Can you work these out from the model? Positions are in its coordinate system, mm. A direction names the side the tool comes from. Give positions to 0.01 mm unless a question says otherwise; leave off trailing zeros. Write each loop counter-clockwise with the first axis right and the second up, starting at its lowest first coordinate (ties: lowest second). Pieces come first, ordered by that corner, then holes.
1. Suppose I cut it at C-C (z = 41.5). Please give me the cut outline in (x, y), and give its area (3 significant figures).
2. Suppose I cut it at D-D (z = 60.5). Please give me the cut outline in (x, y).
3. If I drill on probe 1 along Z at (x, y) = (0, 6); probe 2 along Y at (x, z) = (0, 47); probe 3 along Z at (x, y) = (-21.5, 4), over which ranges is the centre line in solid material (lowest first)?
4. Thinking about a two-plate mould opening in X: for faces 1 (the flat face through (-1.5, -11, 26)), 2 (the cylindrical face through (-3.34, -25.43, 7.18)), 3 (the cylindrical face through (0.3, 7.57, 11.496)), 4 (the cylindrical face through (0, 7.6, 61.5)), which applies, pulls with the +X half, pulls with the -X half, needs draft (parallel to the pull), parting line crosses it, or undercut?
5. On a 3-axis mill with a long thin cutter (end or side, diameter ignored), from which of +Z, -Z, +X, -X, +Y, -Y can I reach the whole of each face in a straight line? I mean faces 5 (the cylindrical face through (4.5, 8.65, 43.07)), 6 (the cylindrical face through (5.66, 7.94, 12.39)), 7 (the flat face through (1.5, 11, 26)), 8 (the flat face through (0, -9, 25.901)), 9 (the flat face through (-11.95, 0, 27)). Say none if no direction works.
6. Suppose I cut it at B-B (y = 17). Please give me the cut outline in (x, z), and give its area (3 significant figures).
7. I'm going to push flat-ended pins straight in: pin 1 (0.9 mm diameter, centred on x = -0.5, z = 17.5, fed in from -Y); pin 2 (1.5 mm diameter, centred on x = 0.5, z = 26.5, fed in from +Y); pin 3 (10 mm diameter, centred on y = 13.5, z = 20.5, fed in from -X). Where does each tip first touch, or does it pass through?
8. Suppose I cut it at A-A (x = 22.5). Please give me the cut outline in (y, z).
Solid Edge part; units mm, degrees
sketch "Sketch1" plane through (0, 0, 0) normal (0, 0, 1) x (1, 0, 0)
  circle A0 centre (0, 0) radius 9.75
extrude "ProtrusioneEstrusa_1" add sketch "Sketch1" along normal blind 67
sketch "Sketch2" plane through (0, 0, 6.1) normal (0, 0, -1) x (1, 0, 0)
  circle A0 centre (0, 0) radius 25.65
extrude "ProtrusioneEstrusa_2" add sketch "Sketch2" against normal blind 2.2
sketch "Sketch3" plane through (0, 0, 16.6) normal (0, 0, 1) x (1, 0, 0)
  circle A0 centre (0, 0) radius 25.65
extrude "ProtrusioneEstrusa_3" add sketch "Sketch3" along normal blind 3.2
sketch "Sketch4" plane through (0, 0, 19.8) normal (0, 0, 1) x (1, 0, 0)
  line L0 (-11.95, -1.5) -> (-9.6339, -1.5)
  line L1 (-9.6339, -1.5) -> (-9.6339, 1.5)
  line L2 (-11.95, 1.5) -> (-9.6339, 1.5)
  line L3 (-11.95, 0) -> (-11.95, 1.5)
  line L4 (-11.95, 0) -> (-11.95, -1.5)
  line L5 (0, -11.95) -> (1.5, -11.95)
  line L6 (1.5, -11.95) -> (1.5, -9.6339)
  line L7 (1.5, -9.6339) -> (-1.5, -9.6339)
  line L8 (-1.5, -11.95) -> (-1.5, -9.6339)
  line L9 (0, -11.95) -> (-1.5, -11.95)
  line L10 (1.5, 11.95) -> (1.5, 9.6339)
  line L11 (-1.5, 9.6339) -> (1.5, 9.6339)
  line L12 (-1.5, 11.95) -> (-1.5, 9.6339)
  line L13 (0, 11.95) -> (-1.5, 11.95)
  line L14 (0, 11.95) -> (1.5, 11.95)
  line L15 (11.95, 0) -> (11.95, -1.5)
  line L16 (11.95, -1.5) -> (9.6339, -1.5)
  line L17 (9.6339, 1.5) -> (9.6339, -1.5)
  line L18 (11.95, 1.5) -> (9.6339, 1.5)
  line L19 (11.95, 0) -> (11.95, 1.5)
extrude "ProtrusioneEstrusa_4" add sketch "Sketch4" along normal blind 15
sketch "Sketch5" plane through (0, 5.45, 33.5) normal (0, -1, 0) x (0, 0, -1)
  circle A0 centre (21.05, 0) radius 1
  circle A1 centre (-27, 0) radius 1
extrude "ScavoEstrusione_3" cut sketch "Sketch5" against normal blind 12.2631 and the other way blind 0.5254
sketch "Sketch6" plane through (0, 0, 0) normal (0, 0, -1) x (1, 0, 0)
  line L0 (3.6239, 9.0515) -> (3.6239, 6.1055)
  arc A0 (-3.6239, 6.1055) -> (3.6239, 6.1055) centre (0, 0) cw
  line L1 (-3.6239, 9.0515) -> (-3.6239, 6.1055)
  line L2 (-3.6239, 9.0515) -> (3.6239, 9.0515)
extrude "ProtrusioneEstrusa_5" add sketch "Sketch6" along normal blind 6
sketch "Sketch7" plane through (0, 0.3492, 0) normal (0, 0, -1) x (0, -1, 0)
  circle A0 centre (0.3492, 0) radius 10.346
extrude "ProtrusioneEstrusa_6" add sketch "Sketch7" against normal blind 6.5682
sketch "Sketch8" plane through (0, 0, 0) normal (0, 0, 1) x (1, 0, 0)
  line L0 (-1.5, 6.9397) -> (-1.5, 5.45)
  line L1 (-1.5, 5.45) -> (1.5, 5.45)
  line L2 (1.5, 5.45) -> (1.5, 6.9397)
  arc A0 (1.5, 6.9397) -> (-1.5, 6.9397) centre (0, 0) cw
extrude "ScavoEstrusione_1" cut sketch "Sketch8" along normal mid plane 447.4642
fillet "Rotondo_1" radius 1.5 1 edges at (-1.5, -10.792, 34.8)
fillet "Rotondo_2" radius 1.5 1 edges at (1.5, -10.792, 34.8)
fillet "Rotondo_3" radius 1.5 3 edges at (-10.792, -1.5, 34.8) (-1.5, 10.792, 34.8) (10.792, 1.5, 34.8)
fillet "Rotondo_4" radius 1.5 3 edges at (-10.792, 1.5, 34.8) (1.5, 10.792, 34.8) (10.792, -1.5, 34.8)
sketch "Sketch9" plane through (0, 0, 0) normal (0, 0, -1) x (1, 0, 0)
  circle A0 centre (0, 8.7109) radius 1.2
extrude "ScavoEstrusione_5" cut sketch "Sketch9" along normal up to vertex (6 mm away) and the other way blind 25.9007
sketch "Sketch10" plane through (0, 0, 8.3) normal (0, 0, 1) x (-1, 0, 0)
  arc A0 (-1.6217, 9.6142) -> (1.6217, 9.6142) centre (0, 0) cw
  line L0 (1.1232, 8.2885) -> (1.6217, 9.6142)
  line L1 (-1.1232, 8.2885) -> (-1.6217, 9.6142)
  arc A1 (1.1232, 8.2885) -> (-1.1232, 8.2885) centre (0, 8.7109) cw
extrude "Cutout1" cut sketch "Sketch10" along normal up to vertex (8.3 mm away)
sketch "Sketch11" plane through (-2.3873, -9.0515, -3) normal (0, -1, 0) x (0, 0, 1)
  line L0 (-3, -3.3873) -> (-3, -1.3873)
  line L1 (-0.9394, -1.7204) -> (-3, -1.3873)
  arc A0 (-0.9394, -1.7204) -> (-0.7687, -1.667) centre (-0.9074, -1.523) ccw
  arc A1 (-0.94, -3.0543) -> (-0.7683, -3.1079) centre (-0.9078, -3.2529) cw
  line L2 (-3, -3.3873) -> (-0.94, -3.0543)
  arc A2 (-0.7687, -1.667) -> (-0.7683, -3.1079) centre (-0.075, -2.3873) cw
extrude "ScavoEstrusione_7" cut sketch "Sketch11" against normal blind 3.9764
Checks:
1. outline: circle Ø19.5 at (0, 0); hole (-1.5, 5.45) - (-1.5, 6.94) arc R7.1 ccw (long way) to (1.5, 6.94) - (1.5, 5.45) - close
1. area: 145 mm2
2. outline: (-1.5, 5.45) - (-1, 5.45) - (-1, 9.7) arc R9.75 ccw (long way) to (1, 9.7) - (1, 5.45) - (1.5, 5.45) - (1.5, 6.94) arc R7.1 cw (long way) to (-1.5, 6.94) - close
3. probe 1: z = 0 to 11.45, 13.45 to 59.5, 61.5 to 67
3. probe 2: y = -9.75 to -7.1, 5.45 to 9.75
3. probe 3: z = 6.1 to 8.3, 16.6 to 19.8
4. face 1: pulls with the -X half
4. face 2: parting line crosses it
4. face 3: undercut
4. face 4: undercut
5. face 5: +Z
5. face 6: none
5. face 7: +Z, +X, +Y
5. face 8: -Z
5. face 9: +Z, -X, +Y, -Y
6. outline: (-19.21, 6.1) - (19.21, 6.1) - (19.21, 8.3) - (-19.21, 8.3) - close; (-19.21, 16.6) - (19.21, 16.6) - (19.21, 19.8) - (-19.21, 19.8) - close
6. area: 207 mm2
7. pin 1: stops at y = -25.65
7. pin 2: stops at y = 11.95
7. pin 3: stops at x = -24.18
8. outline: (-12.32, 6.1) - (12.32, 6.1) - (12.32, 8.3) - (-12.32, 8.3) - close; (-12.32, 16.6) - (12.32, 16.6) - (12.32, 19.8) - (-12.32, 19.8) - close
